Check sheet for the modelled part. Datum: model origin and axes. Units: mm. Face numbers are marked on the shaded views. A direction names the side the tool comes from. Coordinates: 2 decimals unless noted, no trailing zeros. Loops run counter-clockwise (first coordinate to the right, second up) from the corner with the lowest first, then second, coordinate; pieces in that order, holes last. Notation, with made-up numbers: M 31.5,-10.75 L 77.5,-10.75 A8 cw 77.5,-4.75 Z; hole C 11.25,-18.5 d4. An arc over 180 degrees is marked long. Return JSON: item names as keys, results as strings.
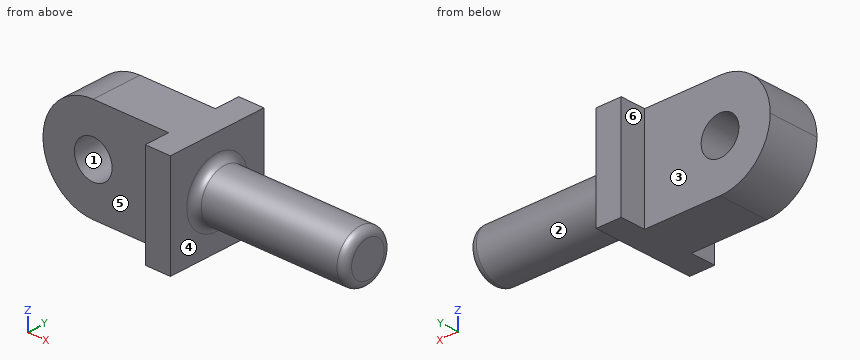
from build123d import *

# Parameters (mm, degrees)
F0_R     = 12.7
F1_DEPTH = 76.2
F3_DEPTH = 25.4
F4_W     = 25.4
F4_H     = 50.8
F5_DEPTH = 63.5
F7_DEPTH = 38.101
F6_R     = 9.525
F8_DEPTH = 38.101
F9_R     = 3.81


with BuildPart() as f1:
    # F0 (on Right) → F1 (new body)
    with BuildSketch(Plane.YZ):
        Circle(F0_R)
    extrude(amount=F1_DEPTH)

    # F2 (on Front) → F3 (join, symmetric)
    with BuildSketch(Plane.XZ):
        Polygon((0, -25.4), (0, 0), (0, 25.4), (-12.7, 25.4), (-12.7, -25.4), align=None)
    extrude(amount=F3_DEPTH, both=True)

    # F4 (on face) → F5 (join)
    with BuildSketch(Plane(origin=(-12.7, 0, 0), x_dir=(0, -1, 0), z_dir=(-1, 0, 0))):
        Rectangle(F4_W, F4_H)
    extrude(amount=F5_DEPTH)

    # F6 (on face) → F7 (cut, through all)
    with BuildSketch(Plane.XZ.offset(12.7)):
        with BuildLine():
            Line((-76.2, 25.4), (-76.2, 0))
            ThreePointArc((-76.2, 0), (-68.760512, 17.960512), (-50.8, 25.4))
            Line((-50.8, 25.4), (-76.2, 25.4))
        make_face()
        with BuildLine():
            ThreePointArc((-50.8, -25.4), (-68.760512, -17.960512), (-76.2, 0))
            Line((-76.2, 0), (-76.2, -25.4))
            Line((-76.2, -25.4), (-50.8, -25.4))
        make_face()
    extrude(amount=-F7_DEPTH, mode=Mode.SUBTRACT)

    # F6 (on face) → F8 (cut, through all)
    with BuildSketch(Plane.XZ.offset(12.7)):
        with Locations((-50.8, 0)):
            Circle(F6_R)
    extrude(amount=-F8_DEPTH, mode=Mode.SUBTRACT)

    # F9
    f9_edges = [f1.edges().sort_by_distance(p)[0] for p in [
        (76.2, -12.7, 0),
        (0, -12.7, 0),
    ]]
    fillet(f9_edges, radius=F9_R)


solid = f1.part
1) Scan lines: line 1 along Z through (x, y) = (-50, -2); line 2 along Y through (x, z) = (-16, 12); line 3 along X through (y, z) = (-18, -16.5). Record each from-to range of solid material in increasing order. Write a range as [from, to].
Answers:
{"line 1": "[-25.4, -9.49], [9.49, 25.4]", "line 2": "[-12.7, 12.7]", "line 3": "[-12.7, 0]"}
2) Section check A-A on y = 0. Record the cut outline in (x, z) (3 decimals).
Answers:
{"outline": "M -76.2,0 A25.4 ccw -50.8,-25.4 L 0,-25.4 L 0,-16.51 A3.81 cw 3.81,-12.7 L 72.39,-12.7 A3.81 ccw 76.2,-8.89 L 76.2,8.89 A3.81 ccw 72.39,12.7 L 3.81,12.7 A3.81 cw 0,16.51 L 0,25.4 L -50.8,25.4 A25.4 ccw Z; hole C -50.8,0 d19.05"}
3) Section check D-D on x = 44.5. Record the cut outline in (y, z), then the cut area to 3 significant figures.
Answers:
{"outline": "C 0,0 d25.4", "area": "507 mm²"}
4) Set-up check for the marked faces 4, 5 and 6: record each of +Z, -Z, +X, -X, +Y, -Y from which the full face is reachable in a straight line by a thin tool's end or side.
Answers:
{"face 4": "+X", "face 5": "+Z, -Z, -X, -Y", "face 6": "+Z, -Z, -X, +Y"}
5) Draft check along Z on the marked faces 1, 2 and 3. Enter one of: +Z half, -Z half, draft (parallel to the pull), parting line (faces both ways), or undercut.
Answers:
{"face 1": "undercut", "face 2": "parting line", "face 3": "draft"}
6) Section check C-C on y = 22. Record the cut outline in (x, z), then the cut area to 3 significant figures.
Answers:
{"outline": "M -12.7,-25.4 L 0,-25.4 L 0,25.4 L -12.7,25.4 Z", "area": "645 mm²"}
7) Section check B-B on x = -32.5. Record the cut outline in (y, z), then the cut area to 3 significant figures.
Answers:
{"outline": "M -12.7,-25.4 L 12.7,-25.4 L 12.7,25.4 L -12.7,25.4 Z", "area": "1,290 mm²"}
8) Go/stop test with flat-tipped pins: pin 1 Ø10 at (x, z) = (33, 19) entering from -Y; pin 2 Ø1.5 at (y, z) = (17, -8) entering from +X; pin 3 Ø6 at (x, y) = (30.5, 8.5) entering from +Z; pin 4 Ø6 at (x, y) = (54, -10.5) entering from +Z. Record where each tip stops, or that it passes through.
Answers:
{"pin 1": "through", "pin 2": "x = 0", "pin 3": "z = 11.45", "pin 4": "z = 10.25"}
